Input: part model. Units: mm. Frame: model coordinates. A direction names the side the tool comes from. Coordinates: 2 decimals unless noted, no trailing zeros. Loops run counter-clockwise (first coordinate to the right, second up) from the corner with the lowest first, then second, coordinate; pieces in that order, holes last. Notation, with made-up numbers: (-39.75, 69) -> (-30.75, 69) arc R15 cw to (-30.75, 87) -> close; hole circle Ø7 at (-13, 44.5). An arc over 180 degrees is marked (long way). Answer as a JSON object with one key per item and string values.
from build123d import *

# Parameters (mm, degrees)
BOSS_EXTRUDE1_DEPTH = 4
BOSS_EXTRUDE2_DEPTH = 20
SKETCH3_R           = 3
CUT_EXTRUDE1_DEPTH  = 62.345545492
SKETCH4_R           = 5
CUT_EXTRUDE2_DEPTH  = 65.381139123
SKETCH5_R           = 3
CUT_EXTRUDE3_DEPTH  = 81.725682082
SKETCH6_R           = 3
CUT_EXTRUDE4_DEPTH  = 80.48760808
SKETCH7_R           = 3
CUT_EXTRUDE5_DEPTH  = 81.516301651
BOSS_EXTRUDE3_DEPTH = 4
FILLET1_R           = 4
FILLET2_R           = 4


with BuildPart() as part:
    # Sketch1 → Boss-Extrude1 (new body)
    with BuildSketch(Plane.XY):
        with BuildLine():
            Line((0, 0), (0, 4))
            Line((0, 4), (-23.425625842, 44.574374158))
            ThreePointArc((-23.425625842, 44.574374158), (-52.116040952, 32.690415109), (-64, 4))
            Line((-64, 4), (-64, 0))
            Line((-64, 0), (0, 0))
        make_face()
    extrude(amount=-BOSS_EXTRUDE1_DEPTH)

    # Sketch2 → Boss-Extrude2 (add)
    with BuildSketch(Plane(origin=(0, 0, -4), x_dir=(-1, 0, 0), z_dir=(0, 0, -1))):
        with BuildLine():
            Line((64, 4), (35.415278297, 4))
            ThreePointArc((35.415278297, 4), (31.691369061, 6.15), (31.691369061, 10.45))
            Line((31.691369061, 10.45), (14.370860985, 20.45))
            Line((14.370860985, 20.45), (28.140384731, 44.299514723))
            ThreePointArc((28.140384731, 44.299514723), (25.787007804, 44.505601014), (23.425625842, 44.574374158))
            Line((23.425625842, 44.574374158), (0, 4))
            Line((0, 4), (0, 0))
            Line((0, 0), (64, 0))
            Line((64, 0), (64, 4))
        make_face()
    extrude(amount=BOSS_EXTRUDE2_DEPTH)

    # Sketch3 → Cut-Extrude1 (cut, through all)
    with BuildSketch(Plane(origin=(-12.447825, 21.560265344, 0), x_dir=(0.8660254037844387, 0.49999999999999983, 0), z_dir=(-0.49999999999999983, 0.8660254037844387, 0))):
        with Locations(Location((-12.220530687, 14, 0), (0, 0, 180))):
            Circle(SKETCH3_R)
    extrude(amount=-CUT_EXTRUDE1_DEPTH, mode=Mode.SUBTRACT)

    # Sketch4 → Cut-Extrude2 (cut, through all)
    with BuildSketch(Plane(origin=(-10.447825, 18.096163729, 0), x_dir=(-0.8660254037844387, -0.49999999999999983, 0), z_dir=(-0.49999999999999983, 0.8660254037844387, 0))):
        with Locations((12.220530687, -14)):
            Circle(SKETCH4_R)
    extrude(amount=-CUT_EXTRUDE2_DEPTH, mode=Mode.SUBTRACT)

    # Sketch5 → Cut-Extrude3 (cut, through all)
    with BuildSketch(Plane(origin=(-1.923035985, -1.110265344, 0), x_dir=(0, 0, 1), z_dir=(-0.8660254037844386, -0.5000000000000001, 0))):
        with Locations(Location((-14, 34.89565, 0), (0, 0, 270))):
            Circle(SKETCH5_R)
    extrude(amount=-CUT_EXTRUDE3_DEPTH, mode=Mode.SUBTRACT)

    # Sketch6 → Cut-Extrude4 (cut, through all)
    with BuildSketch(Plane(origin=(0, 4, 0), x_dir=(1, 0, 0), z_dir=(0, 1, 0))):
        with Locations(Location((-52, 14, 0), (0, 0, 180))):
            Circle(SKETCH6_R)
    extrude(amount=-CUT_EXTRUDE4_DEPTH, mode=Mode.SUBTRACT)

    # Sketch7 → Cut-Extrude5 (cut, through all)
    with BuildSketch(Plane(origin=(0, 0, -4), x_dir=(-1, 0, 0), z_dir=(0, 0, -1))):
        with Locations((28.031115023, 24.110254038)):
            Circle(SKETCH7_R)
    extrude(amount=-CUT_EXTRUDE5_DEPTH, mode=Mode.SUBTRACT)

    # Sketch8 → Boss-Extrude3 (add)
    with BuildSketch(Plane(origin=(0, 0, 0), x_dir=(1, 0, 0), z_dir=(0, 1, 0))):
        with BuildLine():
            Line((-24.111053364, 24), (-4.111053364, 24))
            Line((-4.111053364, 24), (-4.111053364, 32))
            ThreePointArc((-4.111053364, 32), (-14.111053364, 42), (-24.111053364, 32))
            Line((-24.111053364, 32), (-24.111053364, 24))
        make_face()
    extrude(amount=BOSS_EXTRUDE3_DEPTH)

    # Sketch9 → Cut-Revolve2 (revolve, cut)
    with BuildSketch(Plane.XY.offset(-32), mode=Mode.PRIVATE) as cut_revolve2_sk:
        Polygon((-17.111053364, 0), (-17.111053364, 2), (-19.111053364, 4), (-14.111053364, 4), (-14.111053364, 0), align=None)
    revolve(cut_revolve2_sk.sketch.rotate(Axis((-14.111053364, 4, -32), (0, -1, 0)), 270), axis=Axis((-14.111053364, 4, -32), (0, -1, 0)), mode=Mode.SUBTRACT)

    # Fillet1
    fillet1_edges = [part.edges().sort_by_distance(p)[0] for p in [
        (-24.111053364, 4, -28),
        (-14.111053364, 4, -42),
        (-4.111053364, 4, -28),
    ]]
    fillet(fillet1_edges, radius=FILLET1_R - 0.0001)  # a hair under: the kernel refuses the full size

    # Fillet2
    fillet2_edges = [part.edges().sort_by_distance(p)[0] for p in [
        (-64, 2, 0),
        (0, 2, 0),
        (-11.712812921, 24.287187079, 0),
        (-52.116040952, 32.690415109, 0),
    ]]
    fillet(fillet2_edges, radius=FILLET2_R - 0.0001)  # a hair under: the kernel refuses the full size


solid = part.part
1. Pin query (flat end, axial travel): P1, Ø2, axis at y = 6.5, z = -11, coming from the +X side; P2, Ø6, axis at x = -14.5, z = -28.5, coming from the +Y side; P3, Ø22.5, axis at x = -16.5, y = 28, coming from the -Z side. Return the tip coordinate at first contact, or that it passes through.
Reply:
{"P1": "stops at x = -0.87", "P2": "stops at y = 4", "P3": "stops at z = -24"}
2. Section query B-B (z = -14). Return loops of the section in (x, y), plus the area to 3 significant figures.
Reply:
{"outline": "(-64, 0) -> (-55, 0) -> (-55, 4) -> (-64, 4) -> close; (-49, 0) -> (-19.88, 0) -> (-25.36, 9.49) -> (-23.63, 10.49) -> (-25.63, 13.95) -> (-31.69, 10.45) arc R4.3 cw to (-35.42, 4) -> (-49, 4) -> close; (-28.14, 44.3) -> (-20.87, 31.71) -> (-17.22, 33.82) -> (-23.43, 44.57) arc R40.57 ccw to start; (-20.43, 16.95) -> (-18.43, 13.49) -> (-16.7, 14.49) -> (-8.34, 0) -> (0, 0) -> (0, 4) -> (-14.22, 28.62) -> (-17.87, 26.51) -> (-14.37, 20.45) -> close", "area": "519 mm2"}
3. Line query: line 1 along Z through (x, y) = (-52, 2); line 2 along Y through (x, z) = (-40, -5); line 3 along X through (y, z) = (7, -18). Output: solid intervals per line, ascending.
Reply:
{"line 1": "z = -24 to -17, -11 to 0", "line 2": "y = 0 to 4", "line 3": "x = -31.32 to -21.62, -14.69 to -1.73"}
4. Mould query, pull axis Z, two halves, no side actions, for faces 6 (the face through (-22, 12, -24)), 7 (the face through (-1.141, 2.028, -1.203)), 8 (the face through (-20.97, 12.02, -17.26)). Classes: pulls with the +Z half, pulls with the -Z half, needs draft (parallel to the pull), parting line crosses it, or undercut.
Reply:
{"face 6": "pulls with the -Z half", "face 7": "pulls with the +Z half", "face 8": "undercut"}
5. Section query A-A (z = -6). Return loops of the section in (x, y).
Reply:
{"outline": "(-64, 0) -> (0, 0) -> (0, 4) -> (-23.43, 44.57) arc R40.57 ccw to (-28.14, 44.3) -> (-14.37, 20.45) -> (-31.69, 10.45) arc R4.3 cw to (-35.42, 4) -> (-64, 4) -> close"}
6. Access query for faces 1 (the face through (-22.97, 2.8, -27.94)), 2 (the face through (-14, 4, -26)), 3 (the face through (-31.72, 6.1, -13.86)), 4 (the face through (-25.034, 24.242, -2.028)), 5 (the face through (-5.252, 2.797, -28.056)). Directions: +Z, -Z, +X, -X, +Y, -Y. A direction counts if a zero-diameter tool reaches every point of the face in a straight line with its end or side. Return the directions, or none.
Reply:
{"face 1": "-Z, -X, +Y", "face 2": "-Z, +X, -X, +Y", "face 3": "-Z, -X", "face 4": "+Z, -Z", "face 5": "-Z, +X, +Y"}
